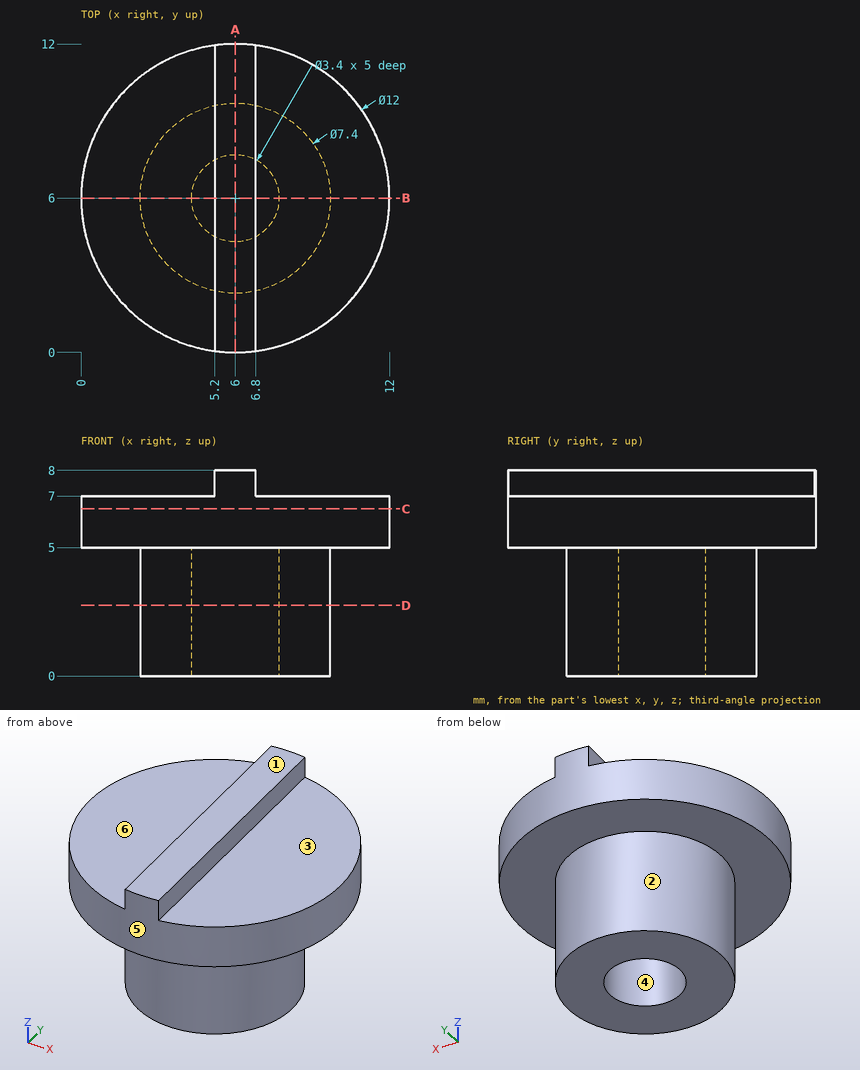
Job drawing, mm, ordinate dimensions from the low corner. One solid piece. A direction names the side the tool comes from. Coordinates: 2 decimals unless noted, no trailing zeros. Order: outer loops, then holes, each group sorted by start corner. A loop starts at its lowest first (then second) coordinate and runs counter-clockwise, first axis right, second up. Notation, with made-up numbers: (69, 61.5) - (115, 61.5) arc R24 cw to (115, 98.5) - close; hole circle Ø9 at (80, 41). An arc over 180 degrees is marked (long way). Return JSON: item names as keys, results as strings. Group by question number.
1) Tool access for the marked faces 1, 2 and 3: list every direction of +Z, -Z, +X, -X, +Y, -Y with a clear straight run to the whole face (end or side of a thin tool).
2) Saw through at A-A, the plane x = 6. Write the cut outline in (y, z).
3) Saw through at C-C, the plane z = 6.5. Write the cut outline in (x, y).
4) Saw through at B-B, the plane y = 6. Write the cut outline in (x, z), plus the area to 3 significant figures.
5) Flat gauge pins, fed straight in: P1, Ø3, axis at x = 6, y = 6, coming from the -Z side; P2, Ø5.5, axis at x = 2, y = 7.5, coming from the +Z side; P3, Ø2, axis at x = 2, z = 2.5, coming from the -Y side. Where does each tip first touch, or does it go through?
6) Saw through at D-D, the plane z = 2.75. Write the cut outline in (x, y).
7) Mould opens along Y. For the marked faces 4, 5 and 6 say: released by +Y, released by -Y, zero draft, split by the parting line, or undercut.
8) Probe line 1 (Y direction, x = 6, z = 3.3); line 2 (Z direction, x = 4, y = 3.5); line 3 (Y direction, x = 4.5, z = 2). List the from-to ranges inside material, lowest first. Write a range as from..to.
Values found:
{
 "1": {"face 1": "+Z, +X, -X, +Y, -Y", "face 2": "-Z", "face 3": "+Z, +X, +Y, -Y"},
 "2": {"outline": "(0, 5) - (2.3, 5) - (2.3, 0) - (4.3, 0) - (4.3, 5) - (7.7, 5) - (7.7, 0) - (9.7, 0) - (9.7, 5) - (12, 5) - (12, 8) - (0, 8) - close"},
 "3": {"outline": "circle Ø12 at (6, 6)"},
 "4": {"outline": "(0, 5) - (2.3, 5) - (2.3, 0) - (4.3, 0) - (4.3, 5) - (7.7, 5) - (7.7, 0) - (9.7, 0) - (9.7, 5) - (12, 5) - (12, 7) - (6.8, 7) - (6.8, 8) - (5.2, 8) - (5.2, 7) - (0, 7) - close", "area": "45.6 mm²"},
 "5": {"P1": "stops at z = 5", "P2": "stops at z = 7", "P3": "stops at y = 3.83"},
 "6": {"outline": "circle Ø7.4 at (6, 6); hole circle Ø3.4 at (6, 6)"},
 "7": {"face 4": "undercut", "face 5": "split by the parting line", "face 6": "zero draft"},
 "8": {"line 1": "y = 2.3..4.3, 7.7..9.7", "line 2": "z = 0..7", "line 3": "y = 2.62..5.2, 6.8..9.38"}
}
